Print and shaded views of the part. All mm, measured from the part's lowest x, y and z. Coordinates: 2 decimals unless noted, no trailing zeros. Loops run counter-clockwise (first coordinate to the right, second up) from the corner with the lowest first, then second, coordinate; pieces in that order, holes last.
1) Saw through at C-C, the plane z = 26. Write the cut outline in (x, y), and give its area (3 significant figures).
2) Saw through at A-A, the plane z = 33. Write the cut outline in (x, y), and give its area (3 significant figures).
3) Saw through at B-B, the plane y = 0.6. Write the cut outline in (x, z), and give its area (3 significant figures).
4) Pin check, flat tips, straight feed: pin 1 Ø1 at (y, z) = (1.5, 18) entering from -X; pin 2 Ø1 at (x, y) = (18, 1) entering from -Z; pin 3 Ø1 at (x, y) = (6.5, 0.5) entering from -Z; pin 4 Ø10 at (x, z) = (12.5, 19) entering from -Y. Stop position of each tip, or through.
5) Saw through at D-D, the plane x = 22. Write the cut outline in (y, z).
6) Wall check: line 1 along X through (y, z) = (1, 31); line 2 along Z through (x, y) = (2.5, 1.95); line 3 along X through (y, z) = (1.7, 16). Give the ranges that are in metal, low to high.
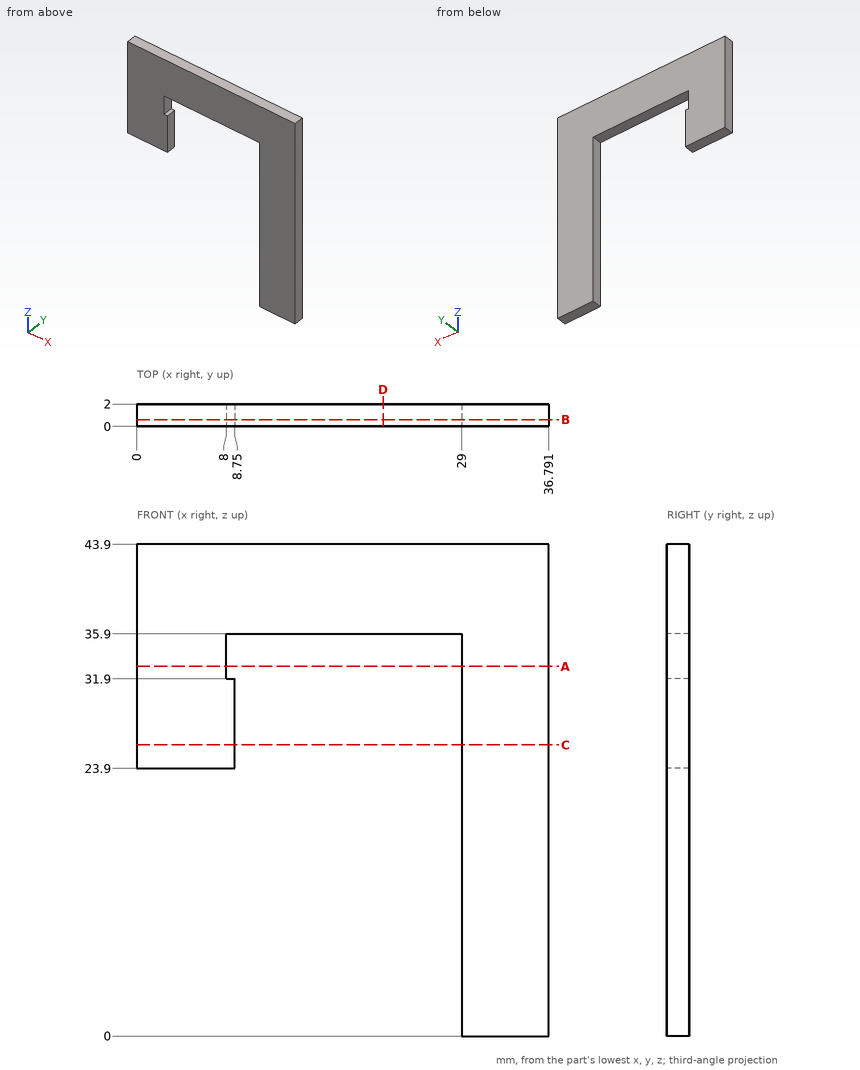
Data:
1. outline: (0, 0) - (8.75, 0) - (8.75, 2) - (0, 2) - close; (29, 0) - (36.79, 0) - (36.79, 2) - (29, 2) - close
1. area: 33.1 mm2
2. outline: (0, 0) - (8, 0) - (8, 2) - (0, 2) - close; (29, 0) - (36.79, 0) - (36.79, 2) - (29, 2) - close
2. area: 31.6 mm2
3. outline: (0, 23.9) - (8.75, 23.9) - (8.75, 31.9) - (8, 31.9) - (8, 35.9) - (29, 35.9) - (29, 0) - (36.79, 0) - (36.79, 43.9) - (0, 43.9) - close
3. area: 676 mm2
4. pin 1: stops at x = 29
4. pin 2: stops at z = 35.9
4. pin 3: stops at z = 23.9
4. pin 4: passes through
5. outline: (0, 35.9) - (2, 35.9) - (2, 43.9) - (0, 43.9) - close
6. line 1: x = 0 to 8.75, 29 to 36.79
6. line 2: z = 23.9 to 43.9
6. line 3: x = 29 to 36.79
